```python
from build123d import *

# Parameters (mm, degrees)
FILLET1_R   = 1.27
HEX_2_DEPTH = 12.573


with BuildPart() as part:
    # BodySke → Base-Revolve (revolve)
    with BuildSketch(Plane.XY, mode=Mode.PRIVATE) as base_revolve_sk:
        Polygon((0, 0), (0, 16.51), (2.54, 19.05), (25.4, 19.05), (25.4, 12.7), (100.33127, 12.7), (101.6, 11.43127), (101.6, 0), align=None)
    revolve(base_revolve_sk.sketch.rotate(Axis((-31.75, 0, 0), (1, 0, 0)), 90), axis=Axis((-31.75, 0, 0), (1, 0, 0)))  # turned: the seam where the file's is

    # Fillet1
    fillet1_edges = [part.edges().sort_by_distance(p)[0] for p in [
        (25.4, 0, -12.7),
    ]]
    fillet(fillet1_edges, radius=FILLET1_R)

    # Sketch2 → Hex-PreBroach (revolve, cut)
    with BuildSketch(Plane.XY, mode=Mode.PRIVATE) as hex_prebroach_sk:
        Polygon((0, 9.525), (12.573, 9.525), (18.072261314, 0), (0, 0), align=None)
    revolve(hex_prebroach_sk.sketch.rotate(Axis((0, 0, 0), (1, 0, 0)), 90), axis=Axis((0, 0, 0), (1, 0, 0)), mode=Mode.SUBTRACT)  # turned: the seam where the file's is

    # Sketch3 → Hex 2 (cut)
    with BuildSketch(Plane(origin=(0, 0, 0), x_dir=(0, 0.5, 0.866025404), z_dir=(-1, 0, 0))):
        Polygon((5.499261314, 9.525), (-5.499261314, 9.525), (-10.998522628, 0), (-5.499261314, -9.525), (5.499261314, -9.525), (10.998522628, 0), align=None)
    extrude(amount=-HEX_2_DEPTH, mode=Mode.SUBTRACT)


solid = part.part
```
Here's how the part is built. I have some questions about the finished solid (model axes, mm). A direction names the side the tool comes from. Round coordinates to 2 decimals unless told otherwise and drop trailing zeros. Order: outer loops, then holes, each group sorted by start corner. A loop starts at its lowest first (then second) coordinate and runs counter-clockwise, first axis right, second up. Notation, with made-up numbers: (52, 14) -> (104, 14) arc R12 ccw to (104, 26) -> close; hole circle Ø5 at (45.25, -6). An arc over 180 degrees is marked (long way). Use a Markdown table: item, result. Add a question column.
(1) For pin 1 Ø3 at (y, z) = (-1.5, -5.5) entering from -X; pin 2 Ø1.4 at (y, z) = (3, -6.5) entering from -X; pin 3 Ø1 at (x, z) = (69, -6.5) entering from +Y, each with a flat end and sliding along its axis, tell me the tip position at first contact or that it passes through.
(2) I need wall thicknesses on line 1 along X through (y, z) = (-3.5, 13.5); line 2 along Y through (x, z) = (72.5, 0.5); line 3 along Y through (x, z) = (8, -7). Which ranges of each line are inside material? Lowest first, please.
(3) Suppose I cut it at A-A, the plane x = 37. Please give me the cut outline in (y, z).
(4) For faces 1 (the face through (25.4, -13, -6)), 2 (the face through (0, 7.1, -7.1)), 3 (the face through (12.573, 5, 9)), which set-ups out of +Z, -Z, +X, -X, +Y, -Y let a thin tool reach every point of the face, with its end or its side?
Verdict:
| question | item | result |
|---|---|---|
| 1 | pin 1 | x = 13.91 |
| 1 | pin 2 | x = 13.53 |
| 1 | pin 3 | y = 11.19 |
| 2 | line 1 | 0 to 25.4 |
| 2 | line 2 | -12.69 to 12.69 |
| 2 | line 3 | -17.72 to -6.96, 6.96 to 17.72 |
| 3 | outline | circle Ø25.4 at (0, 0) |
| 4 | face 1 | +X |
| 4 | face 2 | +Z, -Z, -X, +Y, -Y |
| 4 | face 3 | -X |
